Input: part model. Units: mm. Frame: model coordinates. A direction names the side the tool comes from. Coordinates: 2 decimals unless noted, no trailing zeros. Write each loop counter-clockwise with the first axis right and the second up, starting at its lowest first coordinate (ties: lowest second). Pieces come first, ordered by that corner, then holes.
1) Pin query (flat end, axial travel): pin 1 Ø14.5 at (x, y) = (-76.5, -33.5) entering from +Z; pin 2 Ø4 at (x, y) = (9.5, 23) entering from +Z; pin 3 Ø10 at (x, y) = (65.5, -45) entering from -Z; pin 4 Ø1.5 at (y, z) = (6, 46) entering from -X. Return the tip coordinate at first contact, or that it passes through.
2) Draft query along Y for faces 4 (the cylindrical face through (6, 0, -62)), 5 (the flat face through (0, 0, -80)), 6 (the flat face through (-81.09, -34.04, 0.08)). Return one class per face: pulls with the +Y half, pulls with the -Y half, needs draft (parallel to the pull), parting line crosses it, or undercut.
3) Section query D-D (z = -67.5). Output: boundary loops of the cut face in (x, y).
4) Set-up query: faces 1 (the flat face through (-9.94, 86.46, -0.08)), 2 (the cylindrical face through (-6, 0, -62)), 3 (the flat face through (80, 35, 6)). Return all of +Z, -Z, +X, -X, +Y, -Y with unobstructed straight access to the full face (end or side cutting, diameter ignored); none if empty.
5) Section query A-A (y = 0). Output: boundary loops of the cut face in (x, z), then the cut area to 3 significant figures.
6) Section query B-B (y = 83). State how many separate pieces and enclosed holes the cut face has, then the cut area to 3 significant figures.
7) Line query: L1, parallel to Y at x = 0, z = -4.5; L2, parallel to Y at x = 0, z = 11.5; L3, parallel to Z at x = 69.5, y = 114.5. Output: solid intervals per line, ascending.
from build123d import *

# Parameters (mm, degrees)
SKETCH1_R           = 55
BOSS_EXTRUDE1_DEPTH = 45
SKETCH2_R           = 150
SKETCH2_R_2         = 120
BOSS_EXTRUDE2_DEPTH = 23
BOSS_EXTRUDE3_DEPTH = 6
CIRPATTERN15_COUNT  = 6
FILLET1_R           = 15
BOSS_EXTRUDE4_DEPTH = 35
FILLET2_R           = 10


with BuildPart() as part:
    # Sketch1 → Boss-Extrude1 (new, symmetric)
    with BuildSketch(Plane.XY):
        with Locations(Location((0, 0, 0), (0, 0, 180))):
            Circle(SKETCH1_R)
    extrude(amount=BOSS_EXTRUDE1_DEPTH, both=True)



with BuildPart() as body_2:
    # Sketch2 → Boss-Extrude2 (new, symmetric)
    with BuildSketch(Plane.XY):
        Circle(SKETCH2_R)
        Circle(SKETCH2_R_2, mode=Mode.SUBTRACT)
    extrude(amount=BOSS_EXTRUDE2_DEPTH, both=True)


with BuildPart() as part_1:
    add(part.part)

    add(body_2.part)  # Boss-Extrude3 merges body 2
    # Sketch3 → Boss-Extrude3 (add, symmetric)
    with BuildSketch(Plane.XY):
        with BuildLine():
            Line((-6.292975555, 119.834879975), (-1.690507098, 54.974013732))
            ThreePointArc((-1.690507098, 54.974013732), (-4.686886811, 54.799936971), (-7.669308753, 54.462663387))
            Line((-7.669308753, 54.462663387), (-12.275111778, 119.370522454))
            ThreePointArc((-12.275111778, 119.370522454), (-9.286946418, 119.640096231), (-6.292975555, 119.834879975))
        make_face()
        with BuildLine():
            Line((13.724408526, 119.212585789), (8.33039605, 54.365471594))
            ThreePointArc((8.33039605, 54.365471594), (7.542379524, 54.480386481), (6.752781779, 54.583879839))
            Line((6.752781779, 54.583879839), (12.142889029, 119.38404519))
            ThreePointArc((12.142889029, 119.38404519), (12.933932901, 119.300936206), (13.724408526, 119.212585789))
        make_face()
    boss_extrude3 = extrude(amount=BOSS_EXTRUDE3_DEPTH, both=True)

    # CirPattern15: Boss-Extrude3 ×6 about axis
    cirpattern15_axis = Axis((0, 0, 0), (0, 0, 1))
    for i in range(1, CIRPATTERN15_COUNT):
        add(boss_extrude3.rotate(cirpattern15_axis, i * 360 / CIRPATTERN15_COUNT))

    # Fillet1
    fillet1_edges = [part_1.edges().sort_by_distance(p)[0] for p in [
        (-150, 0, 23),
        (-150, 0, -23),
    ]]
    fillet(fillet1_edges, radius=FILLET1_R)

    # Sketch5 → Boss-Extrude4 (add)
    with BuildSketch(Plane.XY.offset(45)):
        with BuildLine():
            Line((-3.31662479, 5), (3.31662479, 5))
            ThreePointArc((3.31662479, 5), (6, 0), (3.31662479, -5))
            Line((3.31662479, -5), (-3.31662479, -5))
            ThreePointArc((-3.31662479, -5), (-6, 0), (-3.31662479, 5))
        make_face()
    boss_extrude4 = extrude(amount=BOSS_EXTRUDE4_DEPTH)

    # Mirror1: Boss-Extrude4 across plane
    add(boss_extrude4.mirror(Plane.XY))

    # Fillet2
    fillet2_edges = [part_1.edges().sort_by_distance(p)[0] for p in [
        (55, 0, -45),
        (55, 0, 45),
    ]]
    fillet(fillet2_edges, radius=FILLET2_R)


solid = part_1.part
Answer:
1. pin 1: stops at z = 6
1. pin 2: stops at z = 45
1. pin 3: stops at z = -6
1. pin 4: passes through
2. face 4: parting line crosses it
2. face 5: needs draft
2. face 6: undercut
3. outline: (-3.32, -5) - (3.32, -5) arc R6 ccw to (3.32, 5) - (-3.32, 5) arc R6 ccw to start
4. face 1: +Z, -Z
4. face 2: -Z, -X
4. face 3: +Z
5. outline: (-150, -8) arc R15 ccw to (-135, -23) - (-120, -23) - (-120, 23) - (-135, 23) arc R15 ccw to (-150, 8) - close; (-55, -35) arc R10 ccw to (-45, -45) - (-6, -45) - (-6, -80) - (6, -80) - (6, -45) - (45, -45) arc R10 ccw to (55, -35) - (55, 35) arc R10 ccw to (45, 45) - (6, 45) - (6, 80) - (-6, 80) - (-6, 45) - (-45, 45) arc R10 ccw to (-55, 35) - close; (120, -23) - (135, -23) arc R15 ccw to (150, -8) - (150, 8) arc R15 ccw to (135, 23) - (120, 23) - close
5. area: 13,200 mm2
6. separate pieces: 4
6. enclosed holes: 0
6. area: 3,380 mm2
7. L1: y = -150 to -120, -55 to 55, 120 to 150
7. L2: y = -149.59 to -120, -55 to 55, 120 to 149.59
7. L3: z = -23 to 23
